Check sheet for the modelled part. Datum: model origin and axes. Units: mm. A direction names the side the tool comes from. Give positions to 0.01 mm unless a question says otherwise; leave off trailing zeros. Loops run counter-clockwise (first coordinate to the right, second up) from the corner with the lowest first, then second, coordinate; pieces in that order, holes last.
Autodesk Inventor part; units mm, degrees
ref_plane "YZ Plane" through (0, 0, 0) normal (1, 0, 0) x (0, 1, 0)
ref_plane "XZ Plane" through (0, 0, 0) normal (0, 1, 0) x (-1, 0, 0)
ref_plane "XY Plane" through (0, 0, 0) normal (0, 0, 1) x (1, 0, 0)
sketch "Sketch1" plane through (0, 0, 0) normal (0, 1, 0) x (-1, 0, 0)
  line L0 (0, 0) -> (140, 0)
  line L1 (140, 0) -> (140, -120)
  line L2 (140, -120) -> (0, -120)
  line L3 (0, -120) -> (0, 0)
  line L4 (140, 0) -> (0, 0)
  line L5 (0, 0) -> (0, -25)
  line L6 (0, -25) -> (140, -25)
  line L7 (140, -25) -> (140, 0)
  line L8 (140, -120) -> (0, -120)
  line L9 (0, -120) -> (0, -95)
  line L10 (0, -95) -> (140, -95)
  line L11 (140, -95) -> (140, -120)
  line L12 (140, -25) -> (130, -25)
  line L13 (130, -25) -> (130, -95)
  line L14 (130, -95) -> (140, -95)
  line L15 (140, -95) -> (140, -25)
  line L16 (0, -25) -> (10, -25)
  line L17 (10, -25) -> (10, -95)
  line L18 (10, -95) -> (0, -95)
  line L19 (0, -95) -> (0, -25)
  line L20 (130, -25) -> (115, -25)
  line L21 (115, -25) -> (115, -95)
  line L22 (115, -95) -> (130, -95)
  line L23 (130, -95) -> (130, -25)
  line L24 (10, -95) -> (25, -95)
  line L25 (25, -95) -> (25, -25)
  line L26 (25, -25) -> (10, -25)
  line L27 (10, -25) -> (10, -95)
  line L28 (115, -25) -> (25, -25)
  line L29 (25, -25) -> (25, -35)
  line L30 (25, -35) -> (115, -35)
  line L31 (115, -35) -> (115, -25)
  line L32 (115, -95) -> (25, -95)
  line L33 (25, -95) -> (25, -85)
  line L34 (25, -85) -> (115, -85)
  line L35 (115, -85) -> (115, -95)
  line L36 (115, -30) -> (25, -30)
  line L37 (115, -90) -> (25, -90)
  line L38 (115, -30) -> (105, -30)
  line L39 (105, -30) -> (95, -30)
  line L40 (95, -30) -> (85, -30)
  line L41 (85, -30) -> (75, -30)
  line L42 (75, -30) -> (65, -30)
  line L43 (65, -30) -> (55, -30)
  line L44 (55, -30) -> (45, -30)
  line L45 (45, -30) -> (35, -30)
  line L46 (115, -90) -> (105, -90)
  line L47 (105, -90) -> (95, -90)
  line L48 (95, -90) -> (85, -90)
  line L49 (85, -90) -> (75, -90)
  line L50 (75, -90) -> (65, -90)
  line L51 (65, -90) -> (55, -90)
  line L52 (55, -90) -> (45, -90)
  line L53 (45, -90) -> (35, -90)
  line L54 (35, -90) -> (25, -90)
  circle A0 centre (105, -30) radius 1.5
  circle A1 centre (95, -30) radius 1.5
  circle A2 centre (85, -30) radius 1.5
  circle A3 centre (75, -30) radius 1.5
  circle A4 centre (65, -30) radius 1.5
  circle A5 centre (55, -30) radius 1.5
  circle A6 centre (45, -30) radius 1.5
  circle A7 centre (35, -30) radius 1.5
  circle A8 centre (105, -90) radius 1.5
  circle A9 centre (95, -90) radius 1.5
  circle A10 centre (85, -90) radius 1.5
  circle A11 centre (75, -90) radius 1.5
  circle A12 centre (65, -90) radius 1.5
  circle A13 centre (55, -90) radius 1.5
  circle A14 centre (45, -90) radius 1.5
  circle A15 centre (35, -90) radius 1.5
  line L55 (140, 0) -> (105, 0)
  line L56 (105, 0) -> (105, -25)
  line L57 (105, -25) -> (140, -25)
  line L58 (140, -25) -> (140, 0)
  line L59 (140, -95) -> (105, -95)
  line L60 (105, -95) -> (105, -120)
  line L61 (105, -120) -> (140, -120)
  line L62 (140, -120) -> (140, -95)
  line L63 (0, 0) -> (35, 0)
  line L64 (35, 0) -> (35, -25)
  line L65 (35, -25) -> (0, -25)
  line L66 (0, -25) -> (0, 0)
  line L67 (0, -95) -> (35, -95)
  line L68 (35, -95) -> (35, -120)
  line L69 (35, -120) -> (0, -120)
  line L70 (0, -120) -> (0, -95)
  dimension "d0" = 140
  dimension "d1" = 120
  dimension "d2" = 25
  dimension "d3" = 25
  dimension "d4" = 10
  dimension "d5" = 10
  dimension "d6" = 15
  dimension "d7" = 15
  dimension "d8" = 10
  dimension "d9" = 10
  dimension "d10" = 10
  dimension "d11" = 10
  dimension "d12" = 10
  dimension "d13" = 10
  dimension "d14" = 10
  dimension "d15" = 10
  dimension "d16" = 10
  dimension "d17" = 10
  dimension "d18" = 10
  dimension "d19" = 10
  dimension "d20" = 10
  dimension "d21" = 10
  dimension "d22" = 10
  dimension "d23" = 10
  dimension "d24" = 10
  dimension "d25" = 10
  dimension "d26" = 10
  dimension "d27" = 3
  dimension "d28" = 3
  dimension "d29" = 3
  dimension "d30" = 3
  dimension "d31" = 3
  dimension "d32" = 3
  dimension "d33" = 3
  dimension "d34" = 3
  dimension "d35" = 3
  dimension "d36" = 3
  dimension "d37" = 3
  dimension "d38" = 3
  dimension "d39" = 3
  dimension "d40" = 3
  dimension "d41" = 3
  dimension "d42" = 3
  dimension "d43" = 35
  dimension "d44" = 35
  dimension "d45" = 35
  dimension "d46" = 35
extrude "Extrusion1" add sketch "Sketch1" along normal blind 2 contours L0 L64 L6 L3 | L0 L1 L6 L56 | L6 L21 L36 A0 A1 A2 A3 A4 A5 A6 A7 L25 | L10 L68 L2 L3 | L6 L25 L10 L17 | L6 L13 L10 L21 | L36 A7 A6 A5 A4 A3 A2 A1 A0 L21 L30 L25 | L25 L37 A15 A14 A13 A12 A11 A10 A9 A8 L21 L10 | L1 L2 L60 L10 | A7 L36 | L36 A7 | L25 L34 L21 L37 A8 A9 A10 A11 A12 A13 A14 A15 | A0 L36 | L36 A0 | A15 L37 | L37 A15 | A8 L37 | L37 A8
fillet "Fillet1" radius 10 8 edges at (-105, 1, -25) (-115, 1, -85) (-25, 1, -85) (-25, 1, -35) (-115, 1, -35) (-35, 1, -95) (-105, 1, -95) (-35, 1, -25)
sketch "Sketch2" plane through (0, 2, 0) normal (0, 1, 0) x (1, 0, 0)
  line L0 (-130, 95) -> (-130, 25)
  line L1 (-130, 25) -> (-127, 25)
  line L2 (-127, 25) -> (-127, 95)
  line L3 (-127, 95) -> (-130, 95)
  line L4 (-130, 95) -> (-130, 25)
  line L5 (-127, 25) -> (-124.5, 25)
  line L6 (-124.5, 25) -> (-124.5, 95)
  line L7 (-124.5, 95) -> (-127, 95)
  line L8 (-127, 95) -> (-127, 25)
  line L9 (-124.5, 25) -> (-121.5, 25)
  line L10 (-121.5, 25) -> (-121.5, 95)
  line L11 (-121.5, 95) -> (-124.5, 95)
  line L12 (-124.5, 95) -> (-124.5, 25)
  line L13 (-10, 25) -> (-10, 95)
  line L14 (-10, 25) -> (-13, 25)
  line L15 (-13, 25) -> (-13, 95)
  line L16 (-13, 95) -> (-10, 95)
  line L17 (-10, 95) -> (-10, 25)
  line L18 (-13, 25) -> (-15.5, 25)
  line L19 (-15.5, 25) -> (-15.5, 95)
  line L20 (-15.5, 95) -> (-13, 95)
  line L21 (-13, 95) -> (-13, 25)
  line L22 (-15.5, 25) -> (-18.5, 25)
  line L23 (-18.5, 25) -> (-18.5, 95)
  line L24 (-18.5, 95) -> (-15.5, 95)
  line L25 (-15.5, 95) -> (-15.5, 25)
  line L26 (-130, 25) -> (-121.5, 25)
  line L27 (-121.5, 25) -> (-121.5, 35)
  line L28 (-121.5, 35) -> (-130, 35)
  line L29 (-130, 35) -> (-130, 25)
  line L30 (-130, 95) -> (-121.5, 95)
  line L31 (-121.5, 95) -> (-121.5, 85)
  line L32 (-121.5, 85) -> (-130, 85)
  line L33 (-130, 85) -> (-130, 95)
  line L34 (-18.5, 25) -> (-10, 25)
  line L35 (-10, 25) -> (-10, 35)
  line L36 (-10, 35) -> (-18.5, 35)
  line L37 (-18.5, 35) -> (-18.5, 25)
  line L38 (-18.5, 95) -> (-10, 95)
  line L39 (-10, 95) -> (-10, 85)
  line L40 (-10, 85) -> (-18.5, 85)
  line L41 (-18.5, 85) -> (-18.5, 95)
  line L42 (-130, 25) -> (-127, 25)
  line L43 (-127, 25) -> (-127, 35)
  line L44 (-127, 35) -> (-130, 35)
  line L45 (-130, 35) -> (-130, 25)
  line L46 (-18.5, 25) -> (-15.5, 25)
  line L47 (-15.5, 25) -> (-15.5, 35)
  line L48 (-15.5, 35) -> (-18.5, 35)
  line L49 (-18.5, 35) -> (-18.5, 25)
  point P0 (0, 0)
  point P1 (-124.5, 35)
  point P2 (-124.5, 85)
  point P3 (-127, 85)
  point P4 (-13, 35)
  point P5 (-13, 85)
  point P6 (-15.5, 85)
  dimension "d50" = 3
  dimension "d51" = 2.5
  dimension "d52" = 3
  dimension "d53" = 3
  dimension "d54" = 2.5
  dimension "d55" = 3
  dimension "d56" = 10
  dimension "d57" = 10
  dimension "d58" = 10
  dimension "d59" = 10
extrude "Extrusion2" add sketch "Sketch2" along normal blind 5 contours L3 L2 L32 L0 | L28 L2 L1 L0 | L11 L10 L32 L6 | L28 L10 L9 L6 | L14 L15 L36 L13 | L40 L15 L16 L13 | L22 L23 L36 L19 | L40 L23 L24 L19
sketch "Sketch3" plane through (-10, 0, -25) normal (1, 0, 0) x (0, 0, -1)
  line L0 (0, 7) -> (10, 7)
  line L1 (0, 7) -> (2.5, 7)
  line L2 (2.5, 7) -> (2.5, 4.5)
  line L3 (2.5, 4.5) -> (0, 4.5)
  line L4 (0, 4.5) -> (0, 7)
  line L5 (2.5, 4.5) -> (7.5, 4.5)
  circle A0 centre (2.5, 4.5) radius 1
  circle A1 centre (7.5, 4.5) radius 1
  line L6 (60, 7) -> (70, 7)
  line L7 (60, 7) -> (62.5, 7)
  line L8 (62.5, 7) -> (62.5, 4.5)
  line L9 (62.5, 4.5) -> (60, 4.5)
  line L10 (60, 4.5) -> (60, 7)
  line L11 (62.5, 4.5) -> (67.5, 4.5)
  circle A2 centre (67.5, 4.5) radius 1
  circle A3 centre (62.5, 4.5) radius 1
  point P0 (-25, 0)
  dimension "d62" = 2.5
  dimension "d63" = 2.5
  dimension "d64" = 5
  dimension "d65" = 2
  dimension "d66" = 2
  dimension "d67" = 2.5
  dimension "d68" = 2.5
  dimension "d69" = 5
  dimension "d70" = 2
  dimension "d71" = 2
extrude "Extrusion3" cut sketch "Sketch3" against normal up to surface (120 mm away) contours A1 | A0 L5 L2 | L2 L3 A0 | L3 L5 A0 | A2 | A3 L11 L8 | L8 L9 A3 | L9 L11 A3
sketch "Sketch4" plane through (0, 2, 0) normal (0, 1, 0) x (1, 0, 0)
  line L0 (0, 95) -> (0, 120)
  line L1 (0, 120) -> (-35, 120)
  line L2 (-35, 120) -> (-35, 92.5)
  line L3 (-35, 92.5) -> (0, 92.5)
  line L4 (0, 92.5) -> (0, 120)
  line L5 (-35, 0) -> (0, 0)
  line L6 (0, 0) -> (-35, 0)
  line L7 (-35, 0) -> (-35, 27.5)
  line L8 (-35, 27.5) -> (0, 27.5)
  line L9 (0, 27.5) -> (0, 0)
  line L10 (-140, 120) -> (-140, 95)
  line L11 (-140, 120) -> (-105, 120)
  line L12 (-105, 120) -> (-105, 92.5)
  line L13 (-105, 92.5) -> (-140, 92.5)
  line L14 (-140, 92.5) -> (-140, 120)
  line L15 (-140, 0) -> (-105, 0)
  line L16 (-105, 0) -> (-105, 27.5)
  line L17 (-105, 27.5) -> (-140, 27.5)
  line L18 (-140, 27.5) -> (-140, 0)
  circle A0 centre (-105, 27.5) radius 1
  circle A1 centre (-35, 27.5) radius 1
  circle A2 centre (-35, 92.5) radius 1
  circle A3 centre (-105, 92.5) radius 1
  dimension "d74" = 35
  dimension "d75" = 27.5
  dimension "d76" = 35
  dimension "d77" = 27.5
  dimension "d78" = 35
  dimension "d79" = 27.5
  dimension "d80" = 35
  dimension "d81" = 27.5
  dimension "d82" = 2
  dimension "d83" = 2
  dimension "d84" = 2
  dimension "d85" = 2
extrude "Extrusion4" cut sketch "Sketch4" against normal blind 10 contours A2 L2 L3 | L3 L2 A2 | A1 L8 L7 | L7 L8 A1 | A3 L13 L12 | L12 L13 A3 | A0 L17 L16 | L16 L17 A0
properties part number "base"
(1) Gauge pin test, flat ends, axial feed: pin 1 Ø0.9 at (x, y) = (-11.5, 5.5) entering from +Z; pin 2 Ø3 at (y, z) = (4.5, -87.5) entering from +X; pin 3 Ø2.5 at (x, z) = (-105, -92.5) entering from +Y; pin 4 Ø1.2 at (y, z) = (4.5, -92.5) entering from -X. Record the tip position at first contact, or that the pin passes through.
(2) Section check A-A on x = -58. Record the boundary of the cut face in (y, z).
(3) Access from +Z, -Z, +X, -X, +Y, -Y to the whole of each face (thin tool, end or side, straight path). Record for faces 5 (the face through (-38.01, 1.01, -97.85)), 6 (the face through (-128, 4, -85)), 7 (the face through (-13, 4, -90)).
(4) Section check C-C on x = -75. Record the boundary of the cut face in (y, z).
(5) Material ranges on line 1 (Z direction, x = -10.5, y = 4.5); line 2 (Z direction, x = -45, y = 1.05); line 3 (X direction, y = 0.9, z = -92.5), recorded low to high.
(6) Release check for a two-part mould opening along Z. For faces 1 (the face through (-12, 4, -95)), 2 (the face through (-127, 4, -30)), 3 (the face through (-11, 4, -25)), 4 (the face through (-27.85, 1.01, -81.99)) record: pulls with the +Z half, pulls with the -Z half, needs draft (parallel to the pull), parting line crosses it, or undercut.
(7) Section check D-D on z = -30. Give the number of separate pieces and of enclosed holes in the cut face, plus the area to 3 significant figures.
(8) Section check B-B on z = -66. Record the boundary of the cut face in (x, y).
Computed values:
1. pin 1: stops at z = -25
1. pin 2: stops at x = -10
1. pin 3: stops at y = 2
1. pin 4: passes through
2. outline: (0, -95) - (2, -95) - (2, -85) - (0, -85) - close; (0, -35) - (2, -35) - (2, -25) - (0, -25) - close
3. face 5: -Z, +Y, -Y
3. face 6: +X, -X, +Y
3. face 7: +Z, -Z, +Y
4. outline: (0, -95) - (2, -95) - (2, -91.5) - (0, -91.5) - close; (0, -88.5) - (2, -88.5) - (2, -85) - (0, -85) - close; (0, -35) - (2, -35) - (2, -31.5) - (0, -31.5) - close; (0, -28.5) - (2, -28.5) - (2, -25) - (0, -25) - close
5. line 1: z = -95 to -93.5, -91.5 to -88.5, -86.5 to -85, -35 to -33.5, -31.5 to -28.5, -26.5 to -25
5. line 2: z = -95 to -91.5, -88.5 to -85, -35 to -31.5, -28.5 to -25
5. line 3: x = -130 to -106, -104 to -36, -34 to -10
6. face 1: pulls with the -Z half
6. face 2: needs draft
6. face 3: pulls with the +Z half
6. face 4: undercut
7. separate pieces: 7
7. enclosed holes: 0
7. area: 264 mm2
8. outline: (-130, 0) - (-115, 0) - (-115, 2) - (-130, 2) - close; (-25, 0) - (-10, 0) - (-10, 2) - (-25, 2) - close
